Could you check a few things on this model? Use its own coordinates, in mm. A direction names the side the tool comes from. Round coordinates to 2 decimals unless told otherwise and drop trailing zeros. Write each loop counter-clockwise with the first axis right and the second up, starting at its lowest first coordinate (ties: lowest second). Pieces come first, ordered by that corner, then holes. Notation, with made-up numbers: (-29.75, 33.25) -> (20.25, 33.25) arc R15 cw to (20.25, 41.25) -> close; hole circle Ø7 at (32.25, 23.25). An arc over 180 degrees is marked (long way). Return JSON: item names as keys, results as strings.
from build123d import *

# Parameters (mm, degrees)
F0_R     = 38.1
F0_R_2   = 33.3375
F1_DEPTH = 50.8
F3_DEPTH = 12.7
F4_R     = 3.175
F5_DEPTH = 25.4


with BuildPart() as f1:
    # F0 (on Top) → F1 (new body)
    with BuildSketch(Plane.XY):
        Circle(F0_R)
        Circle(F0_R_2, mode=Mode.SUBTRACT)
    extrude(amount=F1_DEPTH)

    # F2 (on Top) → F3 (join)
    with BuildSketch(Plane.XY):
        Polygon((-6.35, 35.346381), (-6.35, 6.35), (-35.763424, 6.35), (-35.763424, -6.35), (-6.35, -6.35), (-6.35, -35.284743), (6.35, -35.284743), (6.35, -6.35), (35.550121, -6.35), (35.550121, 6.35), (6.35, 6.35), (6.35, 35.346381), align=None)
    extrude(amount=F3_DEPTH)

    # F4 (on face) → F5 (cut)
    with BuildSketch(Plane.XY.offset(12.7)):
        with Locations((-19.05, 0)):
            Circle(F4_R)
        with Locations((19.05, 0)):
            Circle(F4_R)
        with Locations((0, 19.05)):
            Circle(F4_R)
        with Locations((0, -19.05)):
            Circle(F4_R)
    extrude(amount=-F5_DEPTH, mode=Mode.SUBTRACT)


solid = f1.part
1) I want a section at A-A, the plane y = 0. Please give me the cut outline in (x, z) (1 decimal), and give its area (3 significant figures).
Return value:
{"outline": "(-38.1, 0) -> (-22.2, 0) -> (-22.2, 12.7) -> (-33.3, 12.7) -> (-33.3, 50.8) -> (-38.1, 50.8) -> close; (-15.9, 0) -> (15.9, 0) -> (15.9, 12.7) -> (-15.9, 12.7) -> close; (22.2, 0) -> (38.1, 0) -> (38.1, 50.8) -> (33.3, 50.8) -> (33.3, 12.7) -> (22.2, 12.7) -> close", "area": "1,170 mm²"}
2) Thinking about a two-plate mould opening in Y: for faces 4 (the face through (-30.235, -23.183, 25.044)), 5 (the face through (3.03, -18.1, 6.44)), 6 (the face through (0, -34, 50.8)), which applies, pulls with the +Y half, pulls with the -Y half, needs draft (parallel to the pull), parting line crosses it, or undercut?
Return value:
{"face 4": "parting line crosses it", "face 5": "undercut", "face 6": "needs draft"}
3) If I drill on probe 1 along Y at (x, z) = (0, 3.5) (3 decimals); probe 2 along Y at (x, z) = (-29.5, 4); probe 3 along X at (y, z) = (-9, 4), over which ranges is the centre line in solid material (lowest first)? Write a range as [from, to].
Return value:
{"probe 1": "[-38.1, -22.225], [-15.875, 15.875], [22.225, 38.1]", "probe 2": "[-24.11, -15.53], [-6.35, 6.35], [15.53, 24.11]", "probe 3": "[-37.02, -32.1], [-6.35, 6.35], [32.1, 37.02]"}
4) I want a section at D-D, the plane x = -19.05. Please give me the cut outline in (y, z) (3 decimals).
Return value:
{"outline": "(-32.996, 0) -> (-27.358, 0) -> (-27.358, 50.8) -> (-32.996, 50.8) -> close; (-6.35, 0) -> (-3.175, 0) -> (-3.175, 12.7) -> (-6.35, 12.7) -> close; (3.175, 0) -> (6.35, 0) -> (6.35, 12.7) -> (3.175, 12.7) -> close; (27.358, 0) -> (32.996, 0) -> (32.996, 50.8) -> (27.358, 50.8) -> close"}
5) For faces 1 (the face through (-3, 0, 12.7)), 2 (the face through (0, 0, 0)), 3 (the face through (6.35, 19, 6)), which set-ups out of +Z, -Z, +X, -X, +Y, -Y let a thin tool reach every point of the face, with its end or its side?
Return value:
{"face 1": "+Z", "face 2": "-Z, +X, -X, +Y, -Y", "face 3": "+Z, -Z"}
6) Will these pins go through, and if not, where does the flat tip stop? pin 1 Ø14 at (x, z) = (14.5, 6.5) entering from -Y; pin 2 Ø6.5 at (x, z) = (25.5, 8.5) entering from +Y; pin 3 Ø14 at (y, z) = (22, 6.5) entering from +X.
Return value:
{"pin 1": "y = -37.35", "pin 2": "y = 30.93", "pin 3": "x = 35.02"}
7) I want a section at C-C, the plane x = 25.5. Please give me the cut outline in (y, z).
Return value:
{"outline": "(-28.31, 0) -> (-21.47, 0) -> (-21.47, 50.8) -> (-28.31, 50.8) -> close; (-6.35, 0) -> (6.35, 0) -> (6.35, 12.7) -> (-6.35, 12.7) -> close; (21.47, 0) -> (28.31, 0) -> (28.31, 50.8) -> (21.47, 50.8) -> close"}
8) I want a section at B-B, the plane z = 4.5. Count the separate pieces of the cut face and the enclosed holes in it, and give its area (3 significant figures).
Return value:
{"separate pieces": "1", "enclosed holes": "8", "area": "2,460 mm²"}
